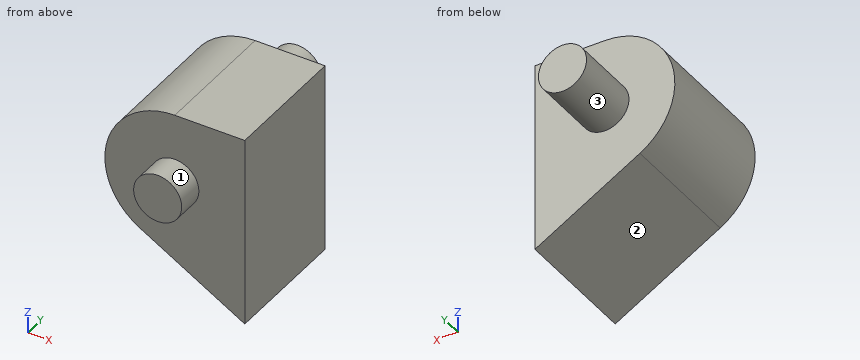
```python
from build123d import *

# Parameters (mm, degrees)
BOSS_EXTRU_1_DEPTH = 14.75
ESQUISSE2_R        = 2.75
BOSS_EXTRU_6_DEPTH = 7.8
BOSS_EXTRU_7_START = -17.9
ESQUISSE2_4_R      = 2.75
BOSS_EXTRU_7_DEPTH = 17.9


with BuildPart() as part:
    # Esquisse1 → Boss.-Extru.1 (new body)
    with BuildSketch(Plane(origin=(0, 0, 0), x_dir=(1, 0, 0), z_dir=(0, 1, 0))):
        with BuildLine():
            Line((0, -8), (8, -8))
            Line((8, -8), (8, 13.856406461))
            Line((8, 13.856406461), (-4, 6.92820323))
            ThreePointArc((-4, 6.92820323), (-7.72740661, -2.070552361), (0, -8))
        make_face()
    extrude(amount=BOSS_EXTRU_1_DEPTH)

    # Esquisse2 → Boss.-Extru.6 (add)
    with BuildSketch(Plane(origin=(0, 14.75, 0), x_dir=(1, 0, 0), z_dir=(0, 1, 0))):
        with Locations(Location((0, 0, 0), (0, 0, 270))):
            Circle(ESQUISSE2_R)
    extrude(amount=BOSS_EXTRU_6_DEPTH)

    # Esquisse2_4 → Boss.-Extru.7 (add)
    with BuildSketch(Plane(origin=(0, 14.75, 0), x_dir=(1, 0, 0), z_dir=(0, 1, 0)).offset(BOSS_EXTRU_7_START)):
        with Locations(Location((0, 0, 0), (0, 0, 270))):
            Circle(ESQUISSE2_4_R)
    extrude(amount=BOSS_EXTRU_7_DEPTH)


solid = part.part
```
Here's how the part is built. I have some questions about the finished solid (model axes, mm). Face numbers are marked on the shaded views. A direction names the side the tool comes from. Coordinates: 2 decimals unless noted, no trailing zeros. Loops run counter-clockwise (first coordinate to the right, second up) from the corner with the lowest first, then second, coordinate; pieces in that order, holes last. Notation, with made-up numbers: (5, 71.25) - (29, 71.25) arc R18 cw to (29, 76.25) - close; hole circle Ø4 at (27.25, 87). An arc over 180 degrees is marked (long way). Return JSON: item names as keys, results as strings. Group by question number.
Item 1: Will these pins go through, and if not, where does the flat tip stop? P1, Ø8, axis at x = -3, y = 16.5, coming from the +Z side; P2, Ø4, axis at y = 4.5, z = -10.5, coming from the -X side; P3, Ø1.5, axis at x = 0, z = -4, coming from the +Y side.
Item 2: If we section it at D-D on y = 17: Write out the boundary of the cut face in (x, z).
Item 3: I need wall thicknesses on line 1 (Y direction, x = -3.5, z = -4); line 2 (X direction, y = -1.75, z = 0); line 3 (Z direction, x = -2, y = 7.75). Which ranges of each line are inside material? Lowest first, please. Write a range as from..to.
Item 4: On a 3-axis mill with a long thin cutter (end or side, diameter ignored), from which of +Z, -Z, +X, -X, +Y, -Y can I reach the whole of each face in a straight line? I mean the marked faces 1, 2 and 3. Say none if no direction works.
Item 5: If we section it at A-A on z = 0: Write out the boundary of the cut face in (x, y).
Item 6: If we section it at B-B on y = 9.5: Write out the boundary of the cut face in (x, z).
Item 7: If we section it at C-C on x = 5: Write out the boundary of the cut face in (y, z), and give its area (3 significant figures).
Calculated:
{
 "1": {"P1": "stops at z = 8", "P2": "stops at x = -1.28", "P3": "stops at y = 14.75"},
 "2": {"outline": "circle Ø5.5 at (0, 0)"},
 "3": {"line 1": "y = 0..14.75", "line 2": "x = -2.75..2.75", "line 3": "z = -8.08..7.75"},
 "4": {"face 1": "-Y", "face 2": "-Z, -X, +Y, -Y", "face 3": "+Y"},
 "5": {"outline": "(-8, 0) - (-2.75, 0) - (-2.75, -3.15) - (2.75, -3.15) - (2.75, 0) - (8, 0) - (8, 14.75) - (2.75, 14.75) - (2.75, 22.55) - (-2.75, 22.55) - (-2.75, 14.75) - (-8, 14.75) - close"},
 "6": {"outline": "(-4, -6.93) - (8, -13.86) - (8, 8) - (0, 8) arc R8 ccw to start"},
 "7": {"outline": "(0, -12.12) - (14.75, -12.12) - (14.75, 8) - (0, 8) - close", "area": "297 mm^2"}
}
